from build123d import *

# Parameters (mm, degrees)
F0_W     = 114.3
F0_H     = 10.7573736592
F0_W_2   = 21.6373776872
F0_H_2   = 16.51
F0_W_3   = 22.1525625052
F1_DEPTH = 152.4
F2_R     = 12.7
F0_H_3   = 22.2626263408
F3_DEPTH = 25.4


with BuildPart() as f1:
    # F0 (on Right) → F1 (new body, symmetric)
    with BuildSketch(Plane.YZ):
        with Locations((0, 11.1313131704)):
            Rectangle(F0_W, F0_H)
        with Locations((92.2932059716, 35.56)):
            Rectangle(F0_W_2, F0_H_2)
        with Locations((-92.0356135626, 35.56)):
            Rectangle(F0_W_3, F0_H_2)
        with BuildLine():
            Line((-57.15, 5.7526263408), (-57.15, 16.51))
            Line((-57.15, 16.51), (-57.15, 35.56))
            ThreePointArc((-57.15, 35.56), (-60.3224589832, 42.164), (-67.4604916954, 43.815))
            Line((-67.4604916954, 43.815), (-80.95933231, 43.815))
            Line((-80.95933231, 43.815), (-80.95933231, 27.305))
            Line((-80.95933231, 27.305), (-57.15, 5.7526263408))
        make_face()
        with BuildLine():
            Line((57.15, 35.56), (57.15, 16.51))
            Line((57.15, 16.51), (57.15, 5.7526263408))
            Line((57.15, 5.7526263408), (81.474517128, 27.305))
            Line((81.474517128, 27.305), (81.474517128, 43.815))
            Line((81.474517128, 43.815), (67.460704078, 43.815))
            ThreePointArc((67.460704078, 43.815), (60.322539648, 42.1640828959), (57.15, 35.56))
        make_face()
        Polygon((-57.15, -16.51), (-57.15, 5.7526263408), (-80.95933231, 27.305), (-103.1118948152, 27.305), align=None)
        Polygon((81.474517128, 27.305), (57.15, 5.7526263408), (57.15, -16.51), (103.1118948152, 27.305), align=None)
    extrude(amount=F1_DEPTH, both=True)

    # F2
    f2_edges = [f1.edges().sort_by_distance(p)[0] for p in [
        (0, -103.111895, 43.815),
        (0, 103.111895, 43.815),
    ]]
    fillet(f2_edges, radius=F2_R)

    # F0 (on Right) + F1_face (on face) + F1_face1 (on face) → F3 (join)
    with BuildSketch(Plane.YZ):
        with Locations((0, 11.1313131704)):
            Rectangle(F0_W, F0_H)
        with BuildLine():
            Line((-57.15, 5.7526263408), (-57.15, 16.51))
            Line((-57.15, 16.51), (-57.15, 35.56))
            ThreePointArc((-57.15, 35.56), (-60.3224589832, 42.164), (-67.4604916954, 43.815))
            Line((-67.4604916954, 43.815), (-80.95933231, 43.815))
            Line((-80.95933231, 43.815), (-80.95933231, 27.305))
            Line((-80.95933231, 27.305), (-57.15, 5.7526263408))
        make_face()
        with BuildLine():
            Line((57.15, 35.56), (57.15, 16.51))
            Line((57.15, 16.51), (57.15, 5.7526263408))
            Line((57.15, 5.7526263408), (81.474517128, 27.305))
            Line((81.474517128, 27.305), (81.474517128, 43.815))
            Line((81.474517128, 43.815), (67.460704078, 43.815))
            ThreePointArc((67.460704078, 43.815), (60.322539648, 42.1640828959), (57.15, 35.56))
        make_face()
        with Locations((0, -5.3786868296)):
            Rectangle(F0_W, F0_H_3)
        Polygon((-57.15, -16.51), (-57.15, 5.7526263408), (-80.95933231, 27.305), (-103.1118948152, 27.305), align=None)
        Polygon((81.474517128, 27.305), (57.15, 5.7526263408), (57.15, -16.51), (103.1118948152, 27.305), align=None)
        with Locations((-92.0356135626, 35.56)):
            Rectangle(F0_W_3, F0_H_2)
        with Locations((92.2932059716, 35.56)):
            Rectangle(F0_W_2, F0_H_2)
    with BuildSketch(Plane(origin=(-152.4, 3.5899e-06, 19.1366208501), x_dir=(0, 1, 0), z_dir=(-1, 0, 0))):
        with BuildLine():
            Line((103.1118912253, -11.9783791499), (103.1118912253, -8.1683791499))
            Line((103.1118912253, -8.1683791499), (57.1499964101, 35.6466208501))
            Line((57.1499964101, 35.6466208501), (57.1499964101, 13.3839945093))
            Line((57.1499964101, 13.3839945093), (-57.1500035899, 13.3839945093))
            Line((-57.1500035899, 13.3839945093), (-57.1500035899, 35.6466208501))
            Line((-57.1500035899, 35.6466208501), (-103.111898405, -8.1683791499))
            Line((-103.111898405, -8.1683791499), (-103.111898405, -11.9783791499))
            ThreePointArc((-103.111898405, -11.9783791499), (-99.3921545261, -20.958635271), (-90.411898405, -24.6783791499))
            Line((-90.411898405, -24.6783791499), (-67.4604952852, -24.6783791499))
            ThreePointArc((-67.4604952852, -24.6783791499), (-60.3224625731, -23.0273791499), (-57.1500035899, -16.4233791499))
            Line((-57.1500035899, -16.4233791499), (-57.1500035899, 2.6266208501))
            Line((-57.1500035899, 2.6266208501), (57.1499964101, 2.6266208501))
            Line((57.1499964101, 2.6266208501), (57.1499964101, -16.4233791499))
            ThreePointArc((57.1499964101, -16.4233791499), (60.3225360581, -23.0274620458), (67.4607004881, -24.6783791499))
            Line((67.4607004881, -24.6783791499), (90.4118912253, -24.6783791499))
            ThreePointArc((90.4118912253, -24.6783791499), (99.3921473464, -20.958635271), (103.1118912253, -11.9783791499))
        make_face()
    with BuildSketch(Plane(origin=(152.4, 3.5899e-06, 19.1366208501), x_dir=(0, 1, 0), z_dir=(1, 0, 0))):
        with BuildLine():
            Line((103.1118912253, 8.1683791499), (103.1118912253, 11.9783791499))
            ThreePointArc((103.1118912253, 11.9783791499), (99.3921473464, 20.958635271), (90.4118912253, 24.6783791499))
            Line((90.4118912253, 24.6783791499), (67.4607004881, 24.6783791499))
            ThreePointArc((67.4607004881, 24.6783791499), (60.3225360581, 23.0274620458), (57.1499964101, 16.4233791499))
            Line((57.1499964101, 16.4233791499), (57.1499964101, -2.6266208501))
            Line((57.1499964101, -2.6266208501), (-57.1500035899, -2.6266208501))
            Line((-57.1500035899, -2.6266208501), (-57.1500035899, 16.4233791499))
            ThreePointArc((-57.1500035899, 16.4233791499), (-60.3224625731, 23.0273791499), (-67.4604952852, 24.6783791499))
            Line((-67.4604952852, 24.6783791499), (-90.411898405, 24.6783791499))
            ThreePointArc((-90.411898405, 24.6783791499), (-99.3921545261, 20.958635271), (-103.111898405, 11.9783791499))
            Line((-103.111898405, 11.9783791499), (-103.111898405, 8.1683791499))
            Line((-103.111898405, 8.1683791499), (-57.1500035899, -35.6466208501))
            Line((-57.1500035899, -35.6466208501), (-57.1500035899, -13.3839945093))
            Line((-57.1500035899, -13.3839945093), (57.1499964101, -13.3839945093))
            Line((57.1499964101, -13.3839945093), (57.1499964101, -35.6466208501))
            Line((57.1499964101, -35.6466208501), (103.1118912253, 8.1683791499))
        make_face()
    extrude(amount=F3_DEPTH, dir=(1, 0, 0))


solid = f1.part
Build history of the part. All positions in model axes, mm. A direction names the side the tool comes from. Round coordinates to 2 decimals unless told otherwise and drop trailing zeros. Write each loop counter-clockwise with the first axis right and the second up, starting at its lowest first coordinate (ties: lowest second). Pieces come first, ordered by that corner, then holes. Notation, with made-up numbers: (58.5, 78) -> (99.5, 78) arc R16 ccw to (99.5, 107) -> close; hole circle Ø6 at (-10, -37). An arc over 180 degrees is marked (long way). Write item = value, one per line.
(1) Band-saw the part on A-A (y = 2). Give the cut face in (x, z), then the cut area to 3 significant figures.
Answer:
outline = (-152.4, 5.75) -> (0, 5.75) -> (0, -16.51) -> (25.4, -16.51) -> (25.4, 5.75) -> (177.8, 5.75) -> (177.8, 16.51) -> (-152.4, 16.51) -> close
area = 4,120 mm2
(2) Band-saw the part on C-C (z = 23.5). Give the cut face in (x, y).
Answer:
outline = (-152.4, -99.12) -> (177.8, -99.12) -> (177.8, -57.15) -> (-152.4, -57.15) -> close; (-152.4, 57.15) -> (177.8, 57.15) -> (177.8, 99.12) -> (-152.4, 99.12) -> close
(3) Tool access for faces 1 (the face through (25.4, -101, 41)), 2 (the face through (-75.133, 99.293, 40.193)), 3 (the face through (103, -1, 5.753)), 4 (the face through (0, -1, -5)), 5 (the face through (10, -57.15, 26)): list every direction of +Z, -Z, +X, -X, +Y, -Y with a clear straight run to the whole face (end or side of a thin tool).
Answer:
face_1 = +Z, +X, -Y
face_2 = +Z, -X, +Y
face_3 = -Z, +X
face_4 = -Z, -X
face_5 = +Z, +X, -X
(4) Band-saw the part on D-D (z = 1). Give the cut face in (x, y), then the cut area to 3 significant figures.
Answer:
outline = (-152.4, -75.52) -> (177.8, -75.52) -> (177.8, -57.15) -> (25.4, -57.15) -> (25.4, 57.15) -> (177.8, 57.15) -> (177.8, 75.52) -> (-152.4, 75.52) -> (-152.4, 57.15) -> (0, 57.15) -> (0, -57.15) -> (-152.4, -57.15) -> close
area = 15,000 mm2
(5) Two-plate mould, pull along Y, no slides. Class faces 6 (the face through (0, 100, 41)), 7 (the face through (13, -103.112, 31)), 8 (the face through (-75, -1, 5.753)): pulls with the +Y half, pulls with the -Y half, needs draft (parallel to the pull), parting line crosses it, or undercut.
Answer:
face_6 = needs draft
face_7 = pulls with the -Y half
face_8 = undercut
(6) Flat gauge pins, fed straight in: pin 1 (10.5 mm diameter, centred on x = -21, y = 89.5, fed in from +Z) (3 decimals); pin 2 (11 mm diameter, centred on x = -83, z = 0, fed in from +Y); pin 3 (6.5 mm diameter, centred on x = -52, z = -4.5, fed in from -Y). Where does each tip first touch, or does it go through?
Answer:
pin_1 = 43.815
pin_2 = 80.24
pin_3 = -73.16
(7) Probe L1, parallel to Y at x = -8, z = 32; L2, parallel to X at y = 52, z = -7.5; L3, parallel to Y at x = 26.5, z = -4.5. List the from-to ranges inside material, lowest first.
Answer:
L1 = -103.08 to -57.15, 57.15 to 103.08
L2 = 0 to 25.4
L3 = -69.75 to -57.15, 57.15 to 69.75
